Could you check a few things on this model? Use its own coordinates, in mm. A direction names the side the tool comes from. Round coordinates to 2 decimals unless told otherwise and drop trailing zeros. Loops run counter-clockwise (first coordinate to the right, second up) from the corner with the lowest first, then second, coordinate; pieces in that order, holes last. Notation, with made-up numbers: (49.5, -28) -> (82.5, -28) arc R16 cw to (82.5, -2) -> close; hole circle Ø4 at (76, -13.75). An arc over 180 degrees is marked (long way). Write each question's results on one line, items separated by ' | '. Start each with the question number.
1) Which directions (+Z, -Z, +X, -X, +Y, -Y) give clear straight access to the entire face, cutting with the end or side of a thin tool? Please do faces 1 (the flat face through (0, -3.5, 40)), 2 (the cylindrical face through (-1.666, -3.993, 74.778)).
2) Imagine slicing it at D-D, the plane x = 0. Give the number of separate pieces and of enclosed holes in the cut face, plus the area to 3 significant figures.
3) We'd pull the mould along X, two halves only. Please class faces 3 (the cylindrical face through (-0.46, 4.01, 47.05)), 4 (the flat face through (-4, 0, 0)), 5 (the flat face through (4.5, 0, 38)): pulls with the +X half, pulls with the -X half, needs draft (parallel to the pull), parting line crosses it, or undercut.
4) If I drill on probe 1 along Z at (x, y) = (0, 4.3); probe 2 along X at (y, z) = (-0.5, 44), over which ranges is the centre line in solid material (lowest first)?
5) Imagine slicing it at B-B, the plane z = 51.5. List the corners of the cut face in (x, y) for me.
6) Imagine slicing it at A-A, the plane y = 1. List the corners of the cut face in (x, z) for me.
7) Imagine slicing it at C-C, the plane z = 34. List the corners of the cut face in (x, y) for me.
8) For P1, Ø2.5, axis at x = 0, z = 73.5, coming from the -Y side; P2, Ø5, axis at x = 0, z = 45, coming from the -Y side, each with a flat end and sliding along its axis, tell me the tip position at first contact or that it passes through.
from build123d import *

# Parameters (mm, degrees)
SKETCH_1_W          = 9
SKETCH_1_H          = 9
EXTRUDE_1_DEPTH     = 78
SKETCH_2_W          = 7
SKETCH_2_H          = 7
CUT_EXTRUDE_1_DEPTH = 78
SKETCH_3_R          = 2.1
CUT_EXTRUDE_2_DEPTH = 75
SKETCH_4_R          = 2.1
CUT_EXTRUDE_3_DEPTH = 75


with BuildPart() as part:
    # ｽｹｯﾁ1 → ﾎﾞｽ - 押し出し1 (new body)
    with BuildSketch(Plane.XY):
        Rectangle(SKETCH_1_W, SKETCH_1_H)
    extrude(amount=EXTRUDE_1_DEPTH)

    # ｽｹｯﾁ2 → ｶｯﾄ - 押し出し1 (cut)
    with BuildSketch(Plane.XY.offset(78)):
        Rectangle(SKETCH_2_W, SKETCH_2_H)
    extrude(amount=-CUT_EXTRUDE_1_DEPTH, mode=Mode.SUBTRACT)

    # ｽｹｯﾁ3 → ｶｯﾄ - 押し出し2 (cut)
    with BuildSketch(Plane(origin=(0, 4.5, 0), x_dir=(1, 0, 0), z_dir=(0, 1, 0))):
        with Locations((0, -4.5)):
            Circle(SKETCH_3_R)
        with Locations((0, -73.5)):
            Circle(SKETCH_3_R)
    extrude(amount=-CUT_EXTRUDE_2_DEPTH, mode=Mode.SUBTRACT)

    # ｽｹｯﾁ4 → ｶｯﾄ - 押し出し3 (cut)
    with BuildSketch(Plane(origin=(0, 4.5, 0), x_dir=(1, 0, 0), z_dir=(0, 1, 0))):
        with Locations((0, -33)):
            Circle(SKETCH_4_R)
        with Locations((0, -45)):
            Circle(SKETCH_4_R)
    extrude(amount=-CUT_EXTRUDE_3_DEPTH, mode=Mode.SUBTRACT)


solid = part.part
Checked values:
1) face 1: +Z, -Z | face 2: +Y, -Y
2) separate pieces: 10 | enclosed holes: 0 | area: 122 mm^2
3) face 3: undercut | face 4: needs draft | face 5: pulls with the +X half
4) probe 1: 0 to 2.4, 6.6 to 30.9, 35.1 to 42.9, 47.1 to 71.4, 75.6 to 78 | probe 2: -4.5 to -3.5, 3.5 to 4.5
5) outline: (-4.5, -4.5) -> (4.5, -4.5) -> (4.5, 4.5) -> (-4.5, 4.5) -> close; hole (-3.5, -3.5) -> (3.5, -3.5) -> (3.5, 3.5) -> (-3.5, 3.5) -> close
6) outline: (-4.5, 0) -> (-3.5, 0) -> (-3.5, 78) -> (-4.5, 78) -> close; (3.5, 0) -> (4.5, 0) -> (4.5, 78) -> (3.5, 78) -> close
7) outline: (-4.5, -4.5) -> (-1.85, -4.5) -> (-1.85, -3.5) -> (-3.5, -3.5) -> (-3.5, 3.5) -> (-1.85, 3.5) -> (-1.85, 4.5) -> (-4.5, 4.5) -> close; (1.85, -4.5) -> (4.5, -4.5) -> (4.5, 4.5) -> (1.85, 4.5) -> (1.85, 3.5) -> (3.5, 3.5) -> (3.5, -3.5) -> (1.85, -3.5) -> close
8) P1: through | P2: y = -4.5
